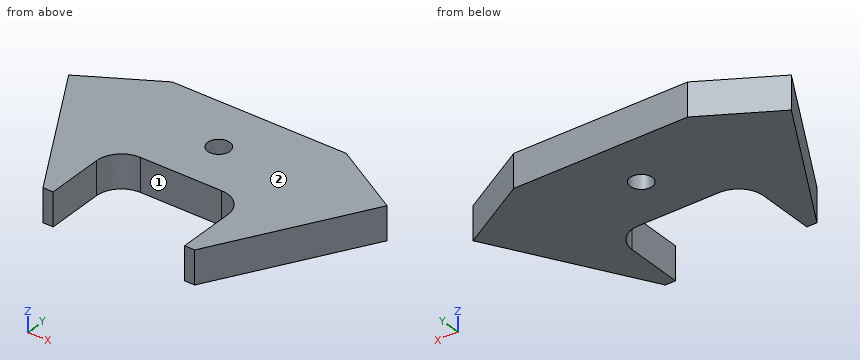
```python
from build123d import *

# Parameters (mm, degrees)
BOSS_EXTRUDE1_DEPTH      = 12.7
FILLET1_R                = 9.525
F_5_16_CLEARANCE_HOLE1_D = 8.4328


with BuildPart() as part:
    # Sketch1 → Boss-Extrude1 (new body)
    with BuildSketch(Plane.XY):
        Polygon((25.019, 0), (28.88945277, 0), (60.63945277, 54.99261314), (33.1431462, 70.86761314), (-33.1431462, 70.86761314), (-60.63945277, 54.99261314), (-28.88945277, 0), (-25.019, 0), (-25.019, 31.369), (25.019, 31.369), align=None)
    extrude(amount=BOSS_EXTRUDE1_DEPTH)

    # Fillet1
    fillet1_edges = [part.edges().sort_by_distance(p)[0] for p in [
        (25.019, 31.369, 6.35),
        (-25.019, 31.369, 6.35),
    ]]
    fillet(fillet1_edges, radius=FILLET1_R)

    # 5/16 Clearance Hole1 (through all)
    with Locations(Plane(origin=(0, 0, 0), x_dir=(-1, 0, 0), z_dir=(0, 0, -1))):
        with Locations((0, 50.419)):
            Hole(F_5_16_CLEARANCE_HOLE1_D / 2)


solid = part.part
```
The model under review builds one solid part; all positions refer to its coordinate system, in mm. Face numbers are marked on the shaded views. A direction names the side the tool comes from. Give positions to 0.01 mm unless a question says otherwise; leave off trailing zeros. Loops run counter-clockwise (first coordinate to the right, second up) from the corner with the lowest first, then second, coordinate; pieces in that order, holes last. Notation, with made-up numbers: (30.5, -37.5) -> (72.5, -37.5) arc R35 ccw to (72.5, 1.5) -> close; hole circle Ø2 at (-9, 88). An arc over 180 degrees is marked (long way). Use CSV: the item, a comma, the result in double quotes.
1. Machinability: for the marked faces 1 and 2, which of the approach directions +Z, -Z, +X, -X, +Y, -Y give a long, thin tool a straight path to every point of the face, cutting with its end or side? Answer none if there is none.
Result:
face 1,"+Z, -Z, -Y"
face 2,"+Z, +X, -X, +Y, -Y"
2. Consider section B-B, the plane y = 53.5. Write out the cut boundary in (x, z).
Result:
outline,"(-59.78, 0) -> (-2.88, 0) -> (-2.88, 12.7) -> (-59.78, 12.7) -> close; (2.88, 0) -> (59.78, 0) -> (59.78, 12.7) -> (2.88, 12.7) -> close"
3. Consider section A-A, the plane x = 0. Write out the cut boundary in (y, z), then the cut area to 3 significant figures.
Result:
outline,"(31.37, 0) -> (46.2, 0) -> (46.2, 12.7) -> (31.37, 12.7) -> close; (54.64, 0) -> (70.87, 0) -> (70.87, 12.7) -> (54.64, 12.7) -> close"
area,"395 mm²"
4. Consider section D-D, the plane x = -32. Write out the cut boundary in (y, z).
Result:
outline,"(5.39, 0) -> (70.87, 0) -> (70.87, 12.7) -> (5.39, 12.7) -> close"
5. For P1, Ø4, axis at y = 23, z = 5, coming from the +X side; P2, Ø1, axis at y = 30.5, z = 3, coming from the +X side; P3, Ø4, axis at y = 45.5, z = 11, coming from the +X side, all flat-tipped, find the tip position at first contact; note any pin that passes through.
Result:
P1,"stops at x = 43.32"
P2,"stops at x = 46.79"
P3,"stops at x = 56.31"
6. To check wall thickness, follow probe 1 along Y at (x, z) = (0, 10); probe 2 along X at (y, z) = (19, 4); probe 3 along X at (y, z) = (4, 9.5). State the ranges of each line that lie inside material, in increasing order. Write a range as from..to.
Result:
probe 1,"y = 31.37..46.2, 54.64..70.87"
probe 2,"x = -39.86..-25.02, 25.02..39.86"
probe 3,"x = -31.2..-25.02, 25.02..31.2"
7. Consider section C-C, the plane z = 8. Write out the cut boundary in (x, y) (3 decimals), then the cut area to 3 significant figures.
Result:
outline,"(-60.639, 54.993) -> (-28.889, 0) -> (-25.019, 0) -> (-25.019, 21.844) arc R9.525 cw to (-15.494, 31.369) -> (15.494, 31.369) arc R9.525 cw to (25.019, 21.844) -> (25.019, 0) -> (28.889, 0) -> (60.639, 54.993) -> (33.143, 70.868) -> (-33.143, 70.868) -> close; hole circle Ø8.433 at (0, 50.419)"
area,"4,830 mm²"
